Can you work these out from the model? Positions are in its coordinate system, mm. Give positions to 0.01 mm unless a question says otherwise; leave off trailing zeros. Answer as a JSON object with one key per item and string values.
```python
from build123d import *

# Parameters (mm, degrees)
F1_DEPTH = 3
F2_DEPTH = 3.5
F3_R     = 1.25
F4_DEPTH = 2
F5_R     = 5.08
F6_R     = 2.54


with BuildPart() as f1:
    # F0 (on Top) → F1 (new body)
    with BuildSketch(Plane.XY):
        Polygon((15, 15), (25, 25), (-25, 25), (-25, -25), (-15, -15), (-15, 15), align=None)
    extrude(amount=F1_DEPTH)

    # F0 (on Top) → F2 (join)
    with BuildSketch(Plane.XY):
        Polygon((-15, -15), (15, 15), (-15, 15), align=None)
    extrude(amount=F2_DEPTH)

    # F3 (on face) → F4 (cut)
    with BuildSketch(Plane.XY.offset(3)):
        with Locations((-20, 20)):
            Circle(F3_R)
        with Locations((0, 20)):
            Circle(F3_R)
        with Locations((-20, 0)):
            Circle(F3_R)
    extrude(amount=-F4_DEPTH, mode=Mode.SUBTRACT)

    # F5
    f5_edges = [f1.edges().sort_by_distance(p)[0] for p in [
        (-25, 25, 1.5),
        (25, 25, 1.5),
        (-25, -25, 1.5),
    ]]
    fillet(f5_edges, radius=F5_R)

    # F6
    f6_edges = [f1.edges().sort_by_distance(p)[0] for p in [
        (-3.592102, 25, 0),
        (17.429103, 21.864032, 0),
        (-23.512102, 23.512102, 0),
        (0, 0, 0),
        (-25, 3.592102, 0),
        (-21.864032, -17.429103, 0),
    ]]
    fillet(f6_edges, radius=F6_R)


solid = f1.part
```
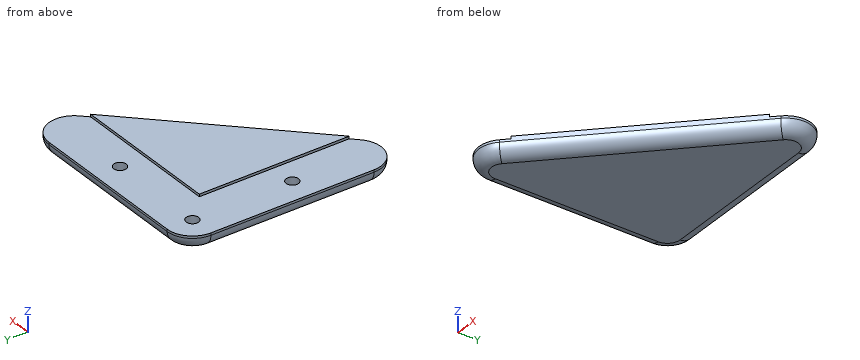
1) Please list where these lines run through material, in increasing order: line 1 along Y through (x, z) = (-20, 1.8); line 2 along X through (y, z) = (-1, 1.1); line 3 along Z through (x, y) = (-17.5, 5.5). Write a range as from..to.
Answer list:
{"line 1": "-17.7..-1.25, 1.25..18.75, 21.25..24.89", "line 2": "-24.55..-20.75, -19.25..-1.63", "line 3": "0..3"}
2) Will these pins go through, and if not, where does the flat tip stop? pin 1 Ø1.5 at (x, z) = (-15, 0.5) entering from +Y; pin 2 Ø1.2 at (x, y) = (-19.5, 0) entering from +Z; pin 3 Ø3 at (x, y) = (-9.5, 19) entering from +Z; pin 4 Ø12 at (x, y) = (2.5, -1.5) entering from +Z.
Answer list:
{"pin 1": "y = 24.65", "pin 2": "z = 1", "pin 3": "z = 3", "pin 4": "z = 3.5"}
3) Suppose I cut it at A-A, the plane z = 1.65. Give the number of separate pieces and of enclosed holes in the cut face, and give its area (3 significant figures).
Answer list:
{"separate pieces": "1", "enclosed holes": "3", "area": "1,140 mm^2"}
